Autodesk Inventor part; units mm, degrees
ref_plane "Work Plane1" through (0, 0, 3.9) normal (0, 0, 1) x (1, 0, 0)
ref_plane "YZ Plane" through (0, 0, 0) normal (1, 0, 0) x (0, 1, 0)
ref_plane "XZ Plane" through (0, 0, 0) normal (0, 1, 0) x (-1, 0, 0)
sketch "Sketch1" plane through (0, 0, 0) normal (0, 1, 0) x (-1, 0, 0)
  circle A0 centre (0, 0) radius 3.9
  dimension "d0" = 7.8
extrude "Extrusion1" add sketch "Sketch1" along normal blind 7
sketch "Sketch5" plane through (0, 0, 0) normal (0, -1, 0) x (1, 0, 0)
  circle A0 centre (0, 0) radius 2.4
  dimension "d22" = 4.8
extrude "Extrusion3" cut sketch "Sketch5" against normal blind 5
ref_plane "Work Plane1" through (0, 0, 3.9) normal (0, 0, 1) x (1, 0, 0)
sketch "Sketch2" plane through (0, 0, 3.9) normal (0, 0, 1) x (1, 0, 0)
  line L0 (0, 0) -> (0, 2.5) construction
  line L1 (3.9, 0) -> (-3.9, 0) construction
  dimension "d21" = 2.5
hole "Hole1" at (0, 2.5, 3.9) direction (0, 0, -1) diameter 2 end through all
properties part number "Lego_Frame_Holder"
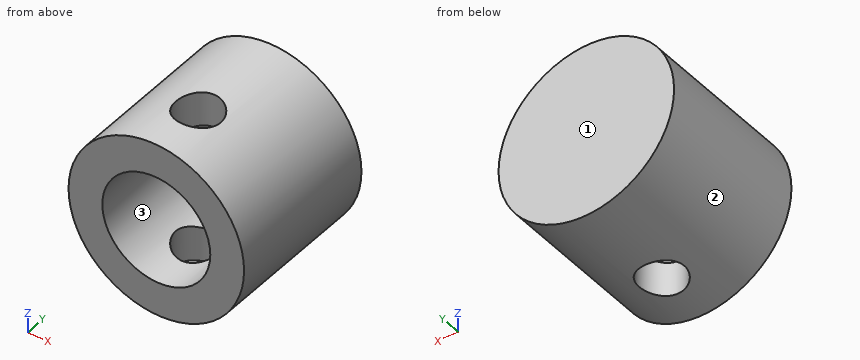
Source: CAD feature listing. Evaluate the final solid. Frame: model axes, mm. Face numbers are marked on the shaded views. Give positions to 0.01 mm unless a question says otherwise; leave off trailing zeros. Loops run counter-clockwise (first coordinate to the right, second up) from the corner with the lowest first, then second, coordinate; pieces in that order, holes last. Notation, with made-up numbers: (1, 70.5) -> (5, 70.5) arc R30 cw to (5, 105.5) -> close; hole circle Ø2 at (67, 26.25). An arc over 180 degrees is marked (long way). Use a Markdown table: item, result. Add a question column.
(1) Section query A-A (x = 0). Output: boundary loops of the cut face in (y, z), then the cut area to 3 significant figures.
(2) Ray query, line 1 (Y direction, x = 0, z = -3.15); line 2 (Z direction, x = 1.25, y = 1.25); line 3 (Z direction, x = 0, y = 3.8). Return the intervals inside material, ascending.
(3) Section query B-B (y = 2). Output: boundary loops of the cut face in (x, z), then the cut area to 3 significant figures.
(4) Pull-direction query (X, two-part tool) for the marked faces 1, 2 and 3; classes: +X half, -X half, draft (parallel to the pull), parting line (faces both ways), or undercut.
(5) Section query C-C (z = 0). Output: boundary loops of the cut face in (x, y).
(6) Section query D-D (x = 2.25). Output: boundary loops of the cut face in (y, z), then the cut area to 3 significant figures.
(7) First-contact query: pin 1 Ø1 at (x, y) = (0.5, 3) entering from -Z; pin 2 Ø2 at (y, z) = (1, 2.5) entering from +X; pin 3 Ø1.5 at (x, y) = (2.5, 4.5) entering from +Z. Flat tips, straight axial feed; report the tip coordinate or a pass-through.
Checked values:
| question | item | result |
|---|---|---|
| 1 | outline | (0, -3.9) -> (1.5, -3.9) -> (1.5, -2.4) -> (0, -2.4) -> close; (0, 2.4) -> (1.5, 2.4) -> (1.5, 3.9) -> (0, 3.9) -> close; (3.5, -3.9) -> (7, -3.9) -> (7, 3.9) -> (3.5, 3.9) -> (3.5, 2.4) -> (5, 2.4) -> (5, -2.4) -> (3.5, -2.4) -> close |
| 1 | area | 24.6 mm^2 |
| 2 | line 1 | 0 to 1.5, 3.5 to 7 |
| 2 | line 2 | -3.69 to -2.05, 2.05 to 3.69 |
| 2 | line 3 | -3.9 to -2.4, 2.4 to 3.9 |
| 3 | outline | (-0.87, -3.8) -> (-0.87, -2.24) arc R2.4 cw to (-0.87, 2.24) -> (-0.87, 3.8) arc R3.9 ccw to start; (0.87, -3.8) arc R3.9 ccw to (0.87, 3.8) -> (0.87, 2.24) arc R2.4 cw to (0.87, -2.24) -> close |
| 3 | area | 24.4 mm^2 |
| 4 | face 1 | draft |
| 4 | face 2 | parting line |
| 4 | face 3 | undercut |
| 5 | outline | (-3.9, 0) -> (-2.4, 0) -> (-2.4, 5) -> (2.4, 5) -> (2.4, 0) -> (3.9, 0) -> (3.9, 7) -> (-3.9, 7) -> close |
| 6 | outline | (0, -3.19) -> (7, -3.19) -> (7, 3.19) -> (0, 3.19) -> (0, 0.84) -> (5, 0.84) -> (5, -0.84) -> (0, -0.84) -> close |
| 6 | area | 36.2 mm^2 |
| 7 | pin 1 | z = -3.89 |
| 7 | pin 2 | x = 3.6 |
| 7 | pin 3 | z = 3.49 |
